from build123d import *

# Parameters (mm, degrees)
F0_W     = 60
F0_H     = 50
F1_DEPTH = 25
F2_R     = 15
F3_DEPTH = 25.001
F4_W     = 7.128705
F4_H     = 9.750254
F5_DEPTH = 25


with BuildPart() as f1:
    # F0 (on Front) → F1 (new body)
    with BuildSketch(Plane.XZ):
        with Locations((30, 25)):
            Rectangle(F0_W, F0_H)
    extrude(amount=F1_DEPTH)

    # F2 (on face) → F3 (cut, through all)
    with BuildSketch(Plane.XZ.offset(25)):
        with Locations((30, 20)):
            Circle(F2_R)
    extrude(amount=-F3_DEPTH, mode=Mode.SUBTRACT)

    # F4 (on face) → F5 (cut)
    with BuildSketch(Plane.XZ.offset(25)):
        with Locations((51.603125, 41.651424)):
            Rectangle(F4_W, F4_H)
    extrude(amount=-F5_DEPTH, mode=Mode.SUBTRACT)


solid = f1.part
Part model, mm, in its own coordinate system. A direction names the side the tool comes from. Give positions to 0.01 mm unless a question says otherwise; leave off trailing zeros. Loops run counter-clockwise (first coordinate to the right, second up) from the corner with the lowest first, then second, coordinate; pieces in that order, holes last. Notation, with made-up numbers: M 72,88 L 117,88 A21 ccw 117,97 Z; hole C -36,71 d8. An arc over 180 degrees is marked long. Put each result on its own line as item: value. Start each with the question number.
1) Saw through at C-C (y = -9.5). List the corners of the cut face in (x, z), then the cut area to 3 significant figures.
2) Probe probe 1 along X at (y, z) = (-1.5, 46); probe 2 along Z at (x, y) = (53, -21); probe 3 along Z at (x, y) = (30, -14.5). List the from-to ranges inside material, lowest first.
3) Pull direction X, two halves, no side cores. Call faces 1 (the flat face through (30, -12, 50)), 2 (the cylindrical face through (26.748, -12.675, 5.357)), 3 (the flat face through (0, -12, 25)): +X half, -X half, draft (parallel to the pull), parting line (faces both ways), or undercut.
4) Flat gauge pin, fed straight in: pin 1 (24 mm diameter, centred on x = 30, z = 20, fed in from -Y). Where does the tip first touch, or does it go through?
5) Saw through at A-A (z = 42). List the corners of the cut face in (x, y), then the cut area to 3 significant figures.
6) Saw through at B-B (x = 30). List the corners of the cut face in (y, z), then the cut area to 3 significant figures.
7) 3-axis set-ups, long thin cutter, end or side, ignore diameter. For faces 4 (the flat face through (60, -12, 25)), 5 (the flat face through (48.039, -13, 42)): which of +Z, -Z, +X, -X, +Y, -Y reach the whole face in a straight line?
Numbers:
1. outline: M 0,0 L 60,0 L 60,50 L 0,50 Z; hole C 30,20 d30; hole M 48.04,36.78 L 55.17,36.78 L 55.17,46.53 L 48.04,46.53 Z
1. area: 2,220 mm^2
2. probe 1: 0 to 48.04, 55.17 to 60
2. probe 2: 0 to 36.78, 46.53 to 50
2. probe 3: 0 to 5, 35 to 50
3. face 1: draft
3. face 2: undercut
3. face 3: -X half
4. pin 1: through
5. outline: M 0,-25 L 48.04,-25 L 48.04,0 L 0,0 Z; M 55.17,-25 L 60,-25 L 60,0 L 55.17,0 Z
5. area: 1,320 mm^2
6. outline: M -25,0 L 0,0 L 0,5 L -25,5 Z; M -25,35 L 0,35 L 0,50 L -25,50 Z
6. area: 500 mm^2
7. face 4: +Z, -Z, +X, +Y, -Y
7. face 5: +Y, -Y
